from build123d import *

# Parameters (mm, degrees)
SKETCH2_W           = 45
SKETCH2_H           = 10
BOSS_EXTRUDE1_DEPTH = 40
SKETCH4_W           = 45
SKETCH4_H           = 10
BOSS_EXTRUDE2_DEPTH = 10
SKETCH8_W           = 45
SKETCH8_H           = 10
BOSS_EXTRUDE3_DEPTH = 20
SKETCH9_R           = 1.45
CUT_EXTRUDE2_DEPTH  = 20
SKETCH10_W          = 45
SKETCH10_H          = 0.626165357
CUT_EXTRUDE3_DEPTH  = 2
SKETCH11_W          = 19
SKETCH11_H          = 42.671327575
BOSS_EXTRUDE4_DEPTH = 1.5
SKETCH12_W          = 13
SKETCH12_H          = 24
BOSS_EXTRUDE5_DEPTH = 1


with BuildPart() as part:
    # Sketch2 → Boss-Extrude1 (new body)
    with BuildSketch(Plane(origin=(0, 0, 0), x_dir=(1, 0, 0), z_dir=(0, 1, 0))):
        Rectangle(SKETCH2_W, SKETCH2_H)
    extrude(amount=BOSS_EXTRUDE1_DEPTH)

    # Sketch4 → Boss-Extrude2 (add)
    with BuildSketch(Plane(origin=(0, 40, 0), x_dir=(1, 0, 0), z_dir=(0, 1, 0))):
        Rectangle(SKETCH4_W, SKETCH4_H)
    extrude(amount=BOSS_EXTRUDE2_DEPTH)

    # Sketch8 → Boss-Extrude3 (add)
    with BuildSketch(Plane.XZ):
        Rectangle(SKETCH8_W, SKETCH8_H)
    extrude(amount=BOSS_EXTRUDE3_DEPTH)

    # Sketch9 → Cut-Extrude2 (cut)
    with BuildSketch(Plane.XY.offset(5)):
        with Locations((19.5, 11.5)):
            Circle(SKETCH9_R)
        with Locations((-19.5, 11.5)):
            Circle(SKETCH9_R)
    extrude(amount=-CUT_EXTRUDE2_DEPTH, mode=Mode.SUBTRACT)

    # Sketch10 → Cut-Extrude3 (cut)
    with BuildSketch(Plane.XY.offset(5)):
        with Locations((0, 22.984410254)):
            Rectangle(SKETCH10_W, SKETCH10_H)
    extrude(amount=-CUT_EXTRUDE3_DEPTH, mode=Mode.SUBTRACT)

    # Sketch11 → Boss-Extrude4 (add)
    with BuildSketch(Plane.XY.offset(5)):
        with Locations((0, 1.335663788)):
            Rectangle(SKETCH11_W, SKETCH11_H)
    extrude(amount=BOSS_EXTRUDE4_DEPTH)

    # Sketch12 → Boss-Extrude5 (add)
    with BuildSketch(Plane.XY.offset(5)):
        with Locations((16, -8)):
            Rectangle(SKETCH12_W, SKETCH12_H)
    extrude(amount=BOSS_EXTRUDE5_DEPTH)


solid = part.part
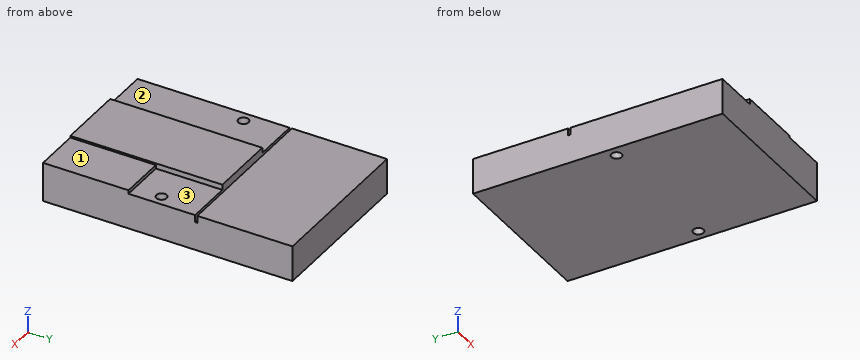
Work out the finished part from the listing and answer in its coordinate system (mm). Face numbers are marked on the shaded views. A direction names the side the tool comes from. Give positions to 0.01 mm unless a question says otherwise; leave off trailing zeros. Loops run counter-clockwise (first coordinate to the right, second up) from the corner with the lowest first, then second, coordinate; pieces in that order, holes last. Notation, with made-up numbers: (-19, -25) - (6, -25) arc R24 cw to (6, -11) - close; hole circle Ø4 at (65.25, 55.5). An arc over 180 degrees is marked (long way). Answer in a Markdown table with one row per item. Add a question column.
Q1. The part is cut by section A-A (x = 19.5). Determine the outline of the cut face in (y, z).
Q2. Consider line 1 along Y through (x, z) = (-19.5, -1.5); line 2 along Y through (x, z) = (-11, 4.75); line 3 along X through (y, z) = (-6, 5.5). Determine where each line is inside the solid, lowest interval first.
Q3. The part is cut by section B-B (y = 11.5). Determine the outline of the cut face in (x, z).
Q4. A tool of negligible diameter and unlimited length cuts with its end or side. For the marked faces 1, 2 and 3, from which of +Z, -Z, +X, -X, +Y, -Y can it reach the whole face along a straight path? Write none if from no direction.
Q5. The part is cut by section C-C (x = -16). Determine the outline of the cut face in (y, z), and give its area (3 significant figures).
Q6. Each of these flat-tipped pins is pushed along its axis until it touches: P1, Ø14.5, axis at x = 17, y = 13.5, coming from the +Z side; P2, Ø2.5, axis at x = 19.5, y = 11.5, coming from the -Z side; P3, Ø6.5, axis at x = 13, y = -10, coming from the +Z side; P4, Ø1.6, axis at y = 9.5, z = 6, coming from the +X side. Where does it stop, or does it pass through?
Q7. The part is cut by section D-D (y = 26.5). Determine the outline of the cut face in (x, z).
Solution:
| question | item | result |
|---|---|---|
| 1 | outline | (-20, -5) - (10.05, -5) - (10.05, 5) - (4, 5) - (4, 6) - (-20, 6) - close; (12.95, -5) - (50, -5) - (50, 5) - (23.3, 5) - (23.3, 3) - (22.67, 3) - (22.67, 5) - (12.95, 5) - close |
| 2 | line 1 | y = -20 to 10.05, 12.95 to 50 |
| 2 | line 2 | y = -20 to 22.67, 23.3 to 50 |
| 2 | line 3 | x = -9.5 to 22.5 |
| 3 | outline | (-22.5, -5) - (-20.95, -5) - (-20.95, 5) - (-22.5, 5) - close; (-18.05, -5) - (18.05, -5) - (18.05, 5) - (9.5, 5) - (9.5, 6.5) - (-9.5, 6.5) - (-9.5, 5) - (-18.05, 5) - close; (20.95, -5) - (22.5, -5) - (22.5, 5) - (20.95, 5) - close |
| 4 | face 1 | +Z, +X, +Y, -Y |
| 4 | face 2 | +Z, -X, +Y, -Y |
| 4 | face 3 | +Z, +X, +Y |
| 5 | outline | (-20, -5) - (50, -5) - (50, 5) - (23.3, 5) - (23.3, 3) - (22.67, 3) - (22.67, 5) - (-20, 5) - close |
| 5 | area | 699 mm² |
| 6 | P1 | stops at z = 5 |
| 6 | P2 | passes through |
| 6 | P3 | stops at z = 6 |
| 6 | P4 | stops at x = 9.5 |
| 7 | outline | (-22.5, -5) - (22.5, -5) - (22.5, 5) - (-22.5, 5) - close |
